Autodesk Inventor part; units mm, degrees
ref_plane "YZ Plane" through (0, 0, 0) normal (1, 0, 0) x (0, 1, 0)
ref_plane "XZ Plane" through (0, 0, 0) normal (0, 1, 0) x (-1, 0, 0)
ref_plane "XY Plane" through (0, 0, 0) normal (0, 0, 1) x (1, 0, 0)
sketch "Sketch1" plane through (0, 0, 0) normal (0, 1, 0) x (-1, 0, 0)
  line L0 (0, 3.2476) -> (0, -3.2476)
  line L1 (0, -3.2476) -> (-1.25, -3.2476)
  line L2 (-1.25, -3.2476) -> (-1.5, -2.9976)
  line L3 (-1.5, -2.9976) -> (-1.5, 2.7524)
  line L4 (-1.5, 2.7524) -> (-2.85, 2.7524)
  line L5 (-2.85, 2.7524) -> (-2.85, 3.0024)
  line L6 (0, 3.2476) -> (-1.1547, 4.4024)
  line L7 (-1.1547, 4.4024) -> (-1.5, 4.4024)
  arc A0 (-1.5, 4.4024) -> (-2.85, 3.0024) centre (0, 1.605) ccw
  line L8 (-1.1547, 4.4024) -> (-0.5774, 5.4024) construction
  line L9 (-0.5774, 5.4024) -> (0.5774, 5.4024) construction
  line L10 (0.5774, 5.4024) -> (1.1547, 4.4024) construction
  line L11 (1.1547, 4.4024) -> (0.5774, 3.4024) construction
  line L12 (0.5774, 3.4024) -> (-0.5774, 3.4024) construction
  line L13 (-0.5774, 3.4024) -> (-1.1547, 4.4024) construction
  point P0 (0, 0)
  point P1 (0, 0)
  point P2 (0, 4.4024)
  dimension "d0" = 3
  dimension "d1" = 6
  dimension "d2" = 0.25
  dimension "d3" = 135
  dimension "d4" = 5.7
  dimension "d5" = 3
  dimension "d6" = 1.65
  dimension "d7" = 2
  dimension "d8" = 0.25
revolve "Revolution1" add sketch "Sketch1" angle 360 about axis through (0, 0, 3.2476) along (0, 0, -1)
sketch "Sketch2" plane through (0, 0, 4.4024) normal (0, 0, 1) x (1, 0, 0)
  circle A0 centre (0, 0) radius 1.1547
  circle A1 centre (0, 0) radius 1.5
  line L0 (-1.1547, 0) -> (-0.5774, 1)
  line L1 (-0.5774, 1) -> (0.5774, 1)
  line L2 (0.5774, 1) -> (1.1547, 0)
  line L3 (1.1547, 0) -> (0.5774, -1)
  line L4 (0.5774, -1) -> (-0.5774, -1)
  line L5 (-0.5774, -1) -> (-1.1547, 0)
  point P0 (0, 0)
extrude "Extrusion1" cut sketch "Sketch2" against normal blind 1.2 contours L3 L4 L5 L0 L1 L2
thread "Thread1"
properties part number "Bolt_M3x0.35_6mm_BH" material "Stainless Steel"
Could you check a few things on this model? Use its own coordinates, in mm. A direction names the side the tool comes from. Coordinates: 2 decimals unless noted, no trailing zeros. Order: outer loops, then holes, each group sorted by start corner. A loop starts at its lowest first (then second) coordinate and runs counter-clockwise, first axis right, second up. Notation, with made-up numbers: M -18,-10 L 3,-10 A35 cw 3,24 Z; hole C 18,-35.75 d2. An arc over 180 degrees is marked long. Use a Markdown table: item, result. Add a question column.
Q1. Which directions (+Z, -Z, +X, -X, +Y, -Y) give clear straight access to the entire face, cutting with the end or side of a thin tool? Please do faces 1 (the flat face through (1.2, 1.2, 2.752)), 2 (the flat face through (0, -1, 4)).
Q2. If I drill on L1, parallel to Z at x = -0.8, y = 0.25; L2, parallel to Y at x = 1.3, z = -0.25; L3, parallel to Z at x = -1.1, y = -0.7, over which ranges is the centre line in solid material (lowest first)?
Q3. We'd pull the mould along X, two halves only. Please class faces 3 (the flat face through (0, 0, -3.248)), 4 (the cylindrical face through (-1.5, 0.07, -0.08)), 5 (the flat face through (0.86, 0.51, 3.81)): pulls with the +X half, pulls with the -X half, needs draft (parallel to the pull), parting line crosses it, or undercut.
Q4. I'm going to push flat-ended pins straight in: pin 1 (3 mm diameter, centred on x = 1, z = -1, fed in from +Y); pin 2 (0.9 mm diameter, centred on x = 0, z = 4, fed in from +Y); pin 3 (0.9 mm diameter, centred on x = 0, z = 3.5, fed in from -Y). Where does each tip first touch, or does it pass through?
Q5. I want a section at A-A on z = -2.25. List the corners of the cut face in (x, y) for me, then the cut area to 3 significant figures.
Checked values:
| question | item | result |
|---|---|---|
| 1 | face 1 | -Z |
| 1 | face 2 | +Z |
| 2 | L1 | -3.25 to 3.2 |
| 2 | L2 | -0.75 to 0.75 |
| 2 | L3 | -3.19 to 4.4 |
| 3 | face 3 | needs draft |
| 3 | face 4 | parting line crosses it |
| 3 | face 5 | undercut |
| 4 | pin 1 | y = 1.5 |
| 4 | pin 2 | y = 2.51 |
| 4 | pin 3 | y = -2.83 |
| 5 | outline | C 0,0 d3 |
| 5 | area | 7.07 mm² |
